For this review, use the dimensioned drawing (mm, ordinates from the lowest corner) and the shaded views. A direction names the side the tool comes from. Round coordinates to 2 decimals unless told otherwise and drop trailing zeros. Loops run counter-clockwise (first coordinate to the right, second up) from the corner with the lowest first, then second, coordinate; pieces in that order, holes last. Notation, with made-up numbers: (81.5, 80.25) - (134.5, 80.25) arc R36 cw to (134.5, 118.25) - close; hole circle Ø9 at (70.25, -6.75). An arc over 180 degrees is marked (long way). Answer as CSV lines item,"result". Start each with the question number.
(1) Wall thickness on L1, parallel to X at y = 121, z = 10 (1 decimal); L2, parallel to Z at x = 10, y = 108 (1 decimal); L3, parallel to Y at x = 79.5, z = 27.5: over which ranges is each line inside the solid? List them lowest first.
(2) Consider section A-A (x = 10.16). Give the boundary of the cut face in (y, z) (1 decimal).
(3) Consider section B-B (z = 10.16). Give the boundary of the cut face in (x, y) (1 decimal), and give its area (3 significant figures).
(4) Consider section C-C (y = 112.5). Count the separate pieces of the cut face and the enclosed holes in it, and give its area (3 significant figures).
(5) For the marked faces 1 and 2, list the 3-axis set-ups (+Z, -Z, +X, -X, +Y, -Y) from which the entire face can be reached by the end or side of a thin tool; tool diameter is ignored.
(6) Consider section D-D (z = 44). Give the boundary of the cut face in (x, y), and give its area (3 significant figures).
(7) For P1, Ø5, axis at x = 42.5, y = 17, coming from the -Z side; P2, Ø4, axis at x = 59, y = 70, coming from the -Z side; P3, Ø1, axis at y = 14, z = 40.5, coming from the -X side, all flat-tipped, find the tip position at first contact; note any pin that passes through.
(8) Mouldability with a two-part tool opening along X and no side actions: class the marked faces 3, 4, 5 and 6 as released by +X, released by -X, zero draft, split by the parting line, or undercut.
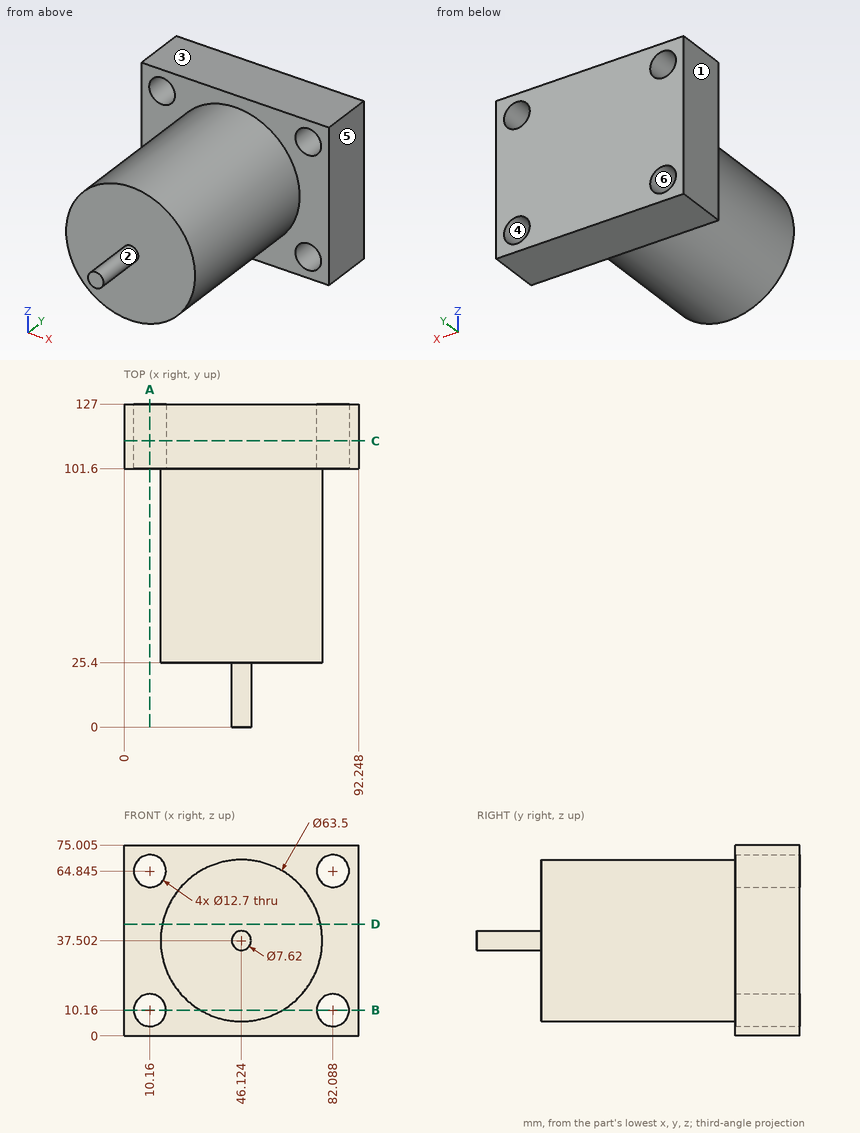
Determined:
1,L1,"x = 0 to 3.8, 16.5 to 75.7, 88.4 to 92.2"
1,L2,"z = 0 to 3.8, 16.5 to 58.5, 71.2 to 75"
1,L3,"y = 101.6 to 127"
2,outline,"(101.6, 0) - (127, 0) - (127, 3.8) - (101.6, 3.8) - close; (101.6, 16.5) - (127, 16.5) - (127, 58.5) - (101.6, 58.5) - close; (101.6, 71.2) - (127, 71.2) - (127, 75) - (101.6, 75) - close"
3,outline,"(0, 101.6) - (3.8, 101.6) - (3.8, 127) - (0, 127) - close; (16.5, 101.6) - (30, 101.6) - (30, 25.4) - (62.3, 25.4) - (62.3, 101.6) - (75.7, 101.6) - (75.7, 127) - (16.5, 127) - close; (88.4, 101.6) - (92.2, 101.6) - (92.2, 127) - (88.4, 127) - close"
3,area,"4,160 mm^2"
4,separate pieces,"1"
4,enclosed holes,"4"
4,area,"6,410 mm^2"
5,face 1,"+Z, -Z, -X, +Y, -Y"
5,face 2,"-Y"
6,outline,"(0, 101.6) - (15.05, 101.6) - (15.05, 25.4) - (77.2, 25.4) - (77.2, 101.6) - (92.25, 101.6) - (92.25, 127) - (0, 127) - close"
6,area,"7,080 mm^2"
7,P1,"stops at z = 33.86"
7,P2,"stops at z = 7.67"
7,P3,"stops at x = 43.25"
8,face 3,"zero draft"
8,face 4,"undercut"
8,face 5,"released by +X"
8,face 6,"undercut"
